```python
from build123d import *

# Parameters (mm, degrees)
PAD_DEPTH       = 10
PAD_DEPTH_BACK  = 8.45
POCKET_DEPTH    = 15.45
SKETCH005_R     = 3
SKETCH005_R_2   = 2.5
PAD001_DEPTH    = 2
SKETCH_R        = 5.75
POCKET002_DEPTH = 5
SKETCH011_W     = 15
SKETCH011_H     = 12
POCKET003_DEPTH = 14
POCKET004_DEPTH = 5
SKETCH013_W     = 11.65
SKETCH013_H     = 6.68
POCKET005_DEPTH = 1.5
SKETCH014_R     = 3.5
POCKET006_DEPTH = 5
SKETCH006_R     = 1
SKETCH006_R_2   = 0.77
SKETCH006_R_3   = 1.125
POCKET009_DEPTH = 2
SKETCH019_W     = 100
SKETCH019_H     = 100
SKETCH019_W_2   = 67
SKETCH019_H_2   = 67.08
POCKET010_DEPTH = 15.5


with BuildPart() as part:
    # Sketch003 → Pad (new body, two sides)
    with BuildSketch(Plane.XZ) as pad_sk:
        Polygon((-35.76, 31.05), (2.39, 31.05), (2.39, 36.05), (14.89, 36.05), (14.89, 31.05), (35.24, 31.05), (35.24, -40.03), (-35.76, -40.03), align=None)
    extrude(amount=PAD_DEPTH)
    extrude(pad_sk.sketch, amount=-PAD_DEPTH_BACK)

    # Sketch004 (on Face9 of Pad) → Pocket (cut)
    with BuildSketch(Plane(origin=(0, 8.45, 0), x_dir=(1, 0, 0), z_dir=(0, 1, 0))):
        Polygon((-33.76, 38.03), (33.24, 38.03), (33.24, -29.05), (12.89, -29.05), (12.89, -34.05), (4.39, -34.05), (4.39, -29.05), (-33.76, -29.05), align=None)
    extrude(amount=-POCKET_DEPTH, mode=Mode.SUBTRACT)

    # Sketch005 (on Face19 of Pocket) → Pad001 (join)
    with BuildSketch(Plane(origin=(0, -7, 0), x_dir=(1, 0, 0), z_dir=(0, 1, 0))):
        with Locations((-4.91, 33.77)):
            Circle(SKETCH005_R)
        with Locations((-29.29, 33.77)):
            Circle(SKETCH005_R)
        with Locations((-29.29, 7.54)):
            Circle(SKETCH005_R)
        with Locations((-4.91, 7.54)):
            Circle(SKETCH005_R)
        with Locations((30.36, 33.28)):
            Circle(SKETCH005_R_2)
        with Locations((18.93, 33.28)):
            Circle(SKETCH005_R_2)
        with Locations((18.55, 16.9)):
            Circle(SKETCH005_R_2)
        with Locations((30.74, 16.9)):
            Circle(SKETCH005_R_2)
        with Locations((28.74, -24.55)):
            Circle(SKETCH005_R)
        with Locations((-29.26, -24.55)):
            Circle(SKETCH005_R)
        with Locations((-29.26, -1.55)):
            Circle(SKETCH005_R)
        with Locations((28.74, -1.55)):
            Circle(SKETCH005_R)
    extrude(amount=PAD001_DEPTH)

    # Sketch → Pocket002 (cut)
    with BuildSketch(Plane(origin=(0, 0, -38.03), x_dir=(-1, 0, 0), z_dir=(0, 0, 1))):
        with Locations((-9.5, -0.098891)):
            Circle(SKETCH_R)
    extrude(amount=-POCKET002_DEPTH, mode=Mode.SUBTRACT)

    # Sketch011 (on Face4 of Pocket002) → Pocket003 (cut)
    with BuildSketch(Plane(origin=(0, 8.45, 0), x_dir=(1, 0, 0), z_dir=(0, 1, 0))):
        with Locations((-33.76, -11.37)):
            Rectangle(SKETCH011_W, SKETCH011_H)
    extrude(amount=-POCKET003_DEPTH, mode=Mode.SUBTRACT)

    # Sketch012 (on Face1 of Pocket003) → Pocket004 (cut)
    with BuildSketch(Plane(origin=(0, 0, 31.05), x_dir=(-1, 0, 0), z_dir=(0, 0, 1))):
        Polygon((-17.41, 1.32), (-25.06, 1.32), (-25.06, 2.98), (-24.11, 4), (-18.36, 4), (-17.41, 2.98), align=None)
    extrude(amount=-POCKET004_DEPTH, mode=Mode.SUBTRACT)

    # Sketch013 (on Face1 of Pocket004) → Pocket005 (cut)
    with BuildSketch(Plane(origin=(0, 0, 31.05), x_dir=(-1, 0, 0), z_dir=(0, 0, 1))):
        with Locations((-21.235, 2.66)):
            Rectangle(SKETCH013_W, SKETCH013_H)
    extrude(amount=-POCKET005_DEPTH, mode=Mode.SUBTRACT)

    # Sketch014 (on Face27 of Pocket005) → Pocket006 (cut)
    with BuildSketch(Plane(origin=(0, -7, 0), x_dir=(1, 0, 0), z_dir=(0, 1, 0))):
        with Locations((7.26, 30.03)):
            Circle(SKETCH014_R)
        with Locations((7.26, 10.03)):
            Circle(SKETCH014_R)
    extrude(amount=-POCKET006_DEPTH, mode=Mode.SUBTRACT)

    # Sketch006 (on Face37 of Pad001) → Pocket009 (cut)
    with BuildSketch(Plane(origin=(0, -5, 0), x_dir=(1, 0, 0), z_dir=(0, 1, 0))):
        with Locations((-29.29, 33.77)):
            Circle(SKETCH006_R)
        with Locations((-4.91, 33.77)):
            Circle(SKETCH006_R)
        with Locations((-4.91, 7.54)):
            Circle(SKETCH006_R)
        with Locations((-29.29, 7.54)):
            Circle(SKETCH006_R)
        with Locations((18.93, 33.28)):
            Circle(SKETCH006_R_2)
        with Locations((30.36, 33.28)):
            Circle(SKETCH006_R_2)
        with Locations((18.55, 16.9)):
            Circle(SKETCH006_R_2)
        with Locations((30.74, 16.9)):
            Circle(SKETCH006_R_2)
        with Locations((-29.26, -1.55)):
            Circle(SKETCH006_R_3)
        with Locations((-29.26, -24.55)):
            Circle(SKETCH006_R_3)
        with Locations((28.74, -24.55)):
            Circle(SKETCH006_R_3)
        with Locations((28.74, -1.55)):
            Circle(SKETCH006_R_3)
    extrude(amount=-POCKET009_DEPTH, mode=Mode.SUBTRACT)

    # Sketch019 (on Face3 of Pocket009) → Pocket010 (cut)
    with BuildSketch(Plane(origin=(0, 8.45, 0), x_dir=(1, 0, 0), z_dir=(0, 1, 0))):
        Rectangle(SKETCH019_W, SKETCH019_H)
        with Locations((-0.26, 4.49)):
            Rectangle(SKETCH019_W_2, SKETCH019_H_2, mode=Mode.SUBTRACT)
    extrude(amount=-POCKET010_DEPTH, mode=Mode.SUBTRACT)


solid = part.part
```
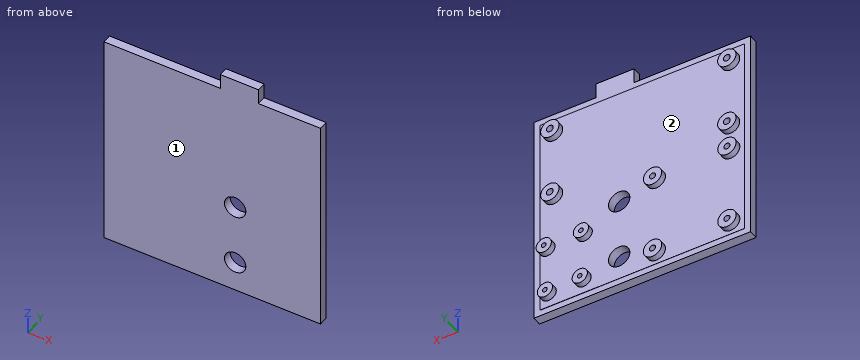
The listing builds one solid part. Answer for the finished solid, in the listing's coordinates (mm). Face numbers are marked on the shaded views. Round coordinates to 2 decimals unless told otherwise and drop trailing zeros. Loops run counter-clockwise (first coordinate to the right, second up) from the corner with the lowest first, then second, coordinate; pieces in that order, holes last.
Q1. For a pull along X with two mould halves and no side action, classify the marked faces 1 and 2 as released by +X, released by -X, zero draft, split by the parting line, or undercut.
Q2. Section C-C, the plane y = -9.25 is taken. Determine the outline of the cut face in (x, z), then the cut area to 3 significant figures.
Q3. Section D-D, the plane z = -3 is taken. Determine the outline of the cut face in (x, y), then the cut area to 3 significant figures.
Q4. Section B-B, the plane x = -4.91 is taken. Determine the outline of the cut face in (y, z), then the cut area to 3 significant figures.
Q5. Given pin 1 Ø3 at (y, z) = (-9, 32.5) entering from -X; pin 2 Ø1.5 at (x, z) = (-19.5, 6.5) entering from +Y, each flat-ended and moving along its own axis, determine where each tip first touches the part or whether it passes through.
Q6. Find the intervals of material crossed by line 1 (Z direction, x = 7.26, y = -7.85); line 2 (X direction, y = -6.4, z = -7.5); line 3 (Z direction, x = -4.91, y = -6.5), in increasing order.
Q7. Section A-A, the plane x = 7.26 is taken. Determine the outline of the cut face in (y, z).
Completed:
1. face 1: zero draft
1. face 2: undercut
2. outline: (-35.76, -40.03) - (35.24, -40.03) - (35.24, 31.05) - (14.89, 31.05) - (14.89, 36.05) - (2.39, 36.05) - (2.39, 31.05) - (-35.76, 31.05) - close; hole circle Ø7 at (7.26, -30.03); hole circle Ø7 at (7.26, -10.03)
2. area: 5,030 mm2
3. outline: (-35.76, -10) - (35.24, -10) - (35.24, -7.05) - (33.24, -7.05) - (33.24, -7) - (-33.76, -7) - (-33.76, -7.05) - (-35.76, -7.05) - close
3. area: 213 mm2
4. outline: (-10, -40.03) - (-7.05, -40.03) - (-7.05, -38.03) - (-7, -38.03) - (-7, -36.77) - (-5, -36.77) - (-5, -34.77) - (-7, -34.77) - (-7, -32.77) - (-5, -32.77) - (-5, -30.77) - (-7, -30.77) - (-7, -10.54) - (-5, -10.54) - (-5, -8.54) - (-7, -8.54) - (-7, -6.54) - (-5, -6.54) - (-5, -4.54) - (-7, -4.54) - (-7, 29.05) - (-7.05, 29.05) - (-7.05, 31.05) - (-10, 31.05) - close
4. area: 229 mm2
5. pin 1: stops at x = -35.76
5. pin 2: stops at y = -7
6. line 1: z = -40.03 to -33.53, -26.53 to -13.53, -6.53 to 36.05
6. line 2: x = -32.29 to -30.29, -28.29 to -26.29, -7.91 to -5.91, -3.91 to -1.91
6. line 3: z = -36.77 to -34.77, -32.77 to -30.77, -10.54 to -8.54, -6.54 to -4.54
7. outline: (-10, -40.03) - (-7.05, -40.03) - (-7.05, -38.03) - (-7, -38.03) - (-7, -33.53) - (-10, -33.53) - close; (-10, -26.53) - (-7, -26.53) - (-7, -13.53) - (-10, -13.53) - close; (-10, -6.53) - (-7, -6.53) - (-7, 29.05) - (-7.05, 29.05) - (-7.05, 36.05) - (-10, 36.05) - close
